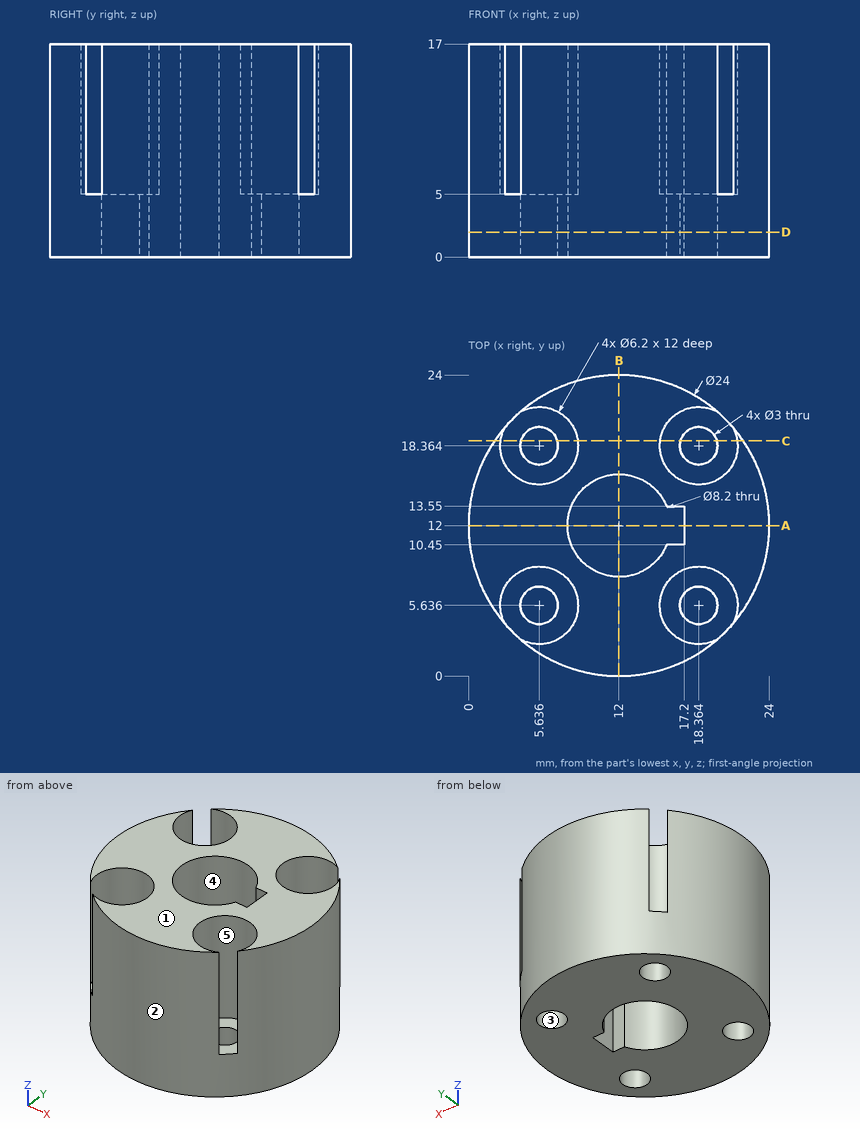
Here's the drawing with two shaded views (mm, measured from the low corner). I have some questions. A direction names the side the tool comes from. Give positions to 0.01 mm unless a question says otherwise; leave off trailing zeros. Write each loop counter-clockwise with the first axis right and the second up, starting at its lowest first coordinate (ties: lowest second). Pieces come first, ordered by that corner, then holes. Notation, with made-up numbers: (-18.75, 19.25) - (12.25, 19.25) arc R16 cw to (12.25, 34.25) - close; hole circle Ø2 at (-26.5, 42.5). An arc over 180 degrees is marked (long way). Write item = value, one per line. Start each with the question number.
1. Imagine slicing it at D-D (z = 2). Please give me the cut outline in (x, y).
2. For pin 1 (5 mm diameter, centred on x = 18.36, y = 5.64, fed in from +Z); pin 2 (8 mm diameter, centred on y = 21, z = 4.5, fed in from -X); pin 3 (1.5 mm diameter, centred on y = 6.5, z = 10.5, fed in from +X), each with a flat end and sliding along its axis, tell me the tip position at first contact or that it passes through.
3. Imagine slicing it at C-C (y = 18.75). Please give me the cut outline in (x, z), and give its area (3 significant figures).
4. On a 3-axis mill with a long thin cutter (end or side, diameter ignored), from which of +Z, -Z, +X, -X, +Y, -Y can I reach the whole of each face in a straight line? I mean the marked faces 4 and 5. Say none if no direction works.
5. Thinking about a two-plate mould opening in X: for the marked faces 1, 2 and 3, which applies, released by +X, released by -X, zero draft, split by the parting line, or undercut?
6. Imagine slicing it at B-B (x = 12). Please give me the cut outline in (y, z).
7. Please list where these lines run through material, in increasing order: line 1 (Y direction, x = 17, z = 14); line 2 (X direction, y = 17.75, z = 2.75); line 3 (Y direction, x = 12, z = 5.25).
8. Imagine slicing it at A-A (y = 12). Please give me the cut outline in (x, z), and give its area (3 significant figures).
Worked answers:
q1.outline = circle Ø24 at (12, 12); hole circle Ø3 at (5.64, 5.64); hole circle Ø3 at (5.64, 18.36); hole (15.8, 10.45) - (17.2, 10.45) - (17.2, 13.55) - (15.8, 13.55) arc R4.1 ccw (long way) to start; hole circle Ø3 at (18.36, 5.64); hole circle Ø3 at (18.36, 18.36)
q2.pin_1 = 5
q2.pin_2 = 1.09
q2.pin_3 = 23.02
q3.outline = (2.08, 0) - (4.19, 0) - (4.19, 5) - (2.56, 5) - (2.56, 17) - (2.08, 17) - close; (7.09, 0) - (16.91, 0) - (16.91, 5) - (15.29, 5) - (15.29, 17) - (8.71, 17) - (8.71, 5) - (7.09, 5) - close; (19.81, 0) - (21.92, 0) - (21.92, 17) - (21.44, 17) - (21.44, 5) - (19.81, 5) - close
q3.area = 161 mm2
q4.face_4 = +Z, -Z
q4.face_5 = +Z
q5.face_1 = zero draft
q5.face_2 = split by the parting line
q5.face_3 = undercut
q6.outline = (0, 0) - (7.9, 0) - (7.9, 17) - (0, 17) - close; (16.1, 0) - (24, 0) - (24, 17) - (16.1, 17) - close
q7.line_1 = 1.09 to 2.85, 8.42 to 10.45, 13.55 to 15.58, 21.15 to 22.91
q7.line_2 = 1.47 to 4.27, 7 to 17, 19.73 to 22.53
q7.line_3 = 0 to 7.9, 16.1 to 24
q8.outline = (0, 0) - (7.9, 0) - (7.9, 17) - (0, 17) - close; (17.2, 0) - (24, 0) - (24, 17) - (17.2, 17) - close
q8.area = 250 mm2
